Read the model definition and answer for the solid it produces. Units are mm, in the model's axes. A direction names the side the tool comes from. Give positions to 0.01 mm unless a question says otherwise; leave off trailing zeros. Order: outer loops, then holes, each group sorted by start corner. A loop starts at its lowest first (then second) coordinate and runs counter-clockwise, first axis right, second up.
Item 1: Given pin 1 Ø3.5 at (y, z) = (-8, 7) entering from -X (3 decimals); pin 2 Ø8 at (y, z) = (22.5, -2.5) entering from -X; pin 3 Ø6 at (y, z) = (-7, 7) entering from +X; pin 4 Ø10 at (x, z) = (-41.5, -6) entering from +Y, each flat-ended and moving along its own axis, determine where each tip first touches the part or whether it passes through.
Item 2: Find the intervals of material crossed by line 1 along Z through (x, y) = (-64, 7); line 2 along X through (y, z) = (-1.5, 8.25) (3 decimals), in increasing order.
Item 3: The mould has two halves that part along Y. Classify faces 3 (the face through (-49, 0, -12.5)), 4 (the face through (-52.461, -14.202, 0.175)), 5 (the face through (-42.024, 24.806, 5.479)): +Y half, -Y half, draft (parallel to the pull), parting line (faces both ways), or undercut.
Item 4: A cutting plane is placed at C-C (z = 1.75). Write down the section's boundary in (x, y) (3 decimals).
Item 5: Which of the six approach directions +Z, -Z, +X, -X, +Y, -Y give full straight-line access (tool end or side, diameter ignored) to faces 1 (the face through (-63.64, -8.52, 8.66)), 2 (the face through (-29, -37.067, 0))?
Item 6: A cutting plane is placed at A-A (z = -7). State how many separate pieces and enclosed holes the cut face has, plus the area to 3 significant figures.
Item 7: A cutting plane is placed at B-B (y = 6). Write down the section's boundary in (x, z) (3 decimals).
Item 8: A cutting plane is placed at D-D (x = -56). Write down the section's boundary in (y, z), plus the area to 3 significant figures.
from build123d import *

# Parameters (mm, degrees)
BOSS_EXTRUDE1_DEPTH     = 12.5
SKETCH3_R               = 2.25
CUT_EXTRUDE1_DEPTH      = 77.872073504
CUT_EXTRUDE2_DEPTH      = 57.106034184
CUT_EXTRUDE2_DEPTH_BACK = 5
SKETCH5_R               = 2.25
FILLET4_R               = 10


with BuildPart() as part:
    # Sketch1 → Boss-Extrude1 (new, symmetric)
    with BuildSketch(Plane.XY):
        with BuildLine():
            Line((-66.175, -12.5), (-66.175, 12.5))
            Line((-66.175, 12.5), (-50.732755691, 12.5))
            ThreePointArc((-50.732755691, 12.5), (-45.469745991, 25.740332157), (-36.825635638, 37.066630004))
            Line((-36.825635638, 37.066630004), (-25.954333745, 37.066630004))
            ThreePointArc((-25.954333745, 37.066630004), (-45.25, 0), (-25.954333745, -37.066630004))
            Line((-25.954333745, -37.066630004), (-36.825635638, -37.066630004))
            ThreePointArc((-36.825635638, -37.066630004), (-45.469745991, -25.740332157), (-50.732755691, -12.5))
            Line((-50.732755691, -12.5), (-66.175, -12.5))
        make_face()
    extrude(amount=BOSS_EXTRUDE1_DEPTH, both=True)

    # Sketch3 → Cut-Extrude1 (cut, symmetric)
    with BuildSketch(Plane(origin=(0, 0, 0), x_dir=(0, 0, 1), z_dir=(-0.8433914458128852, 0.5372996083468248, 0))):
        with Locations(Location((-7, 0, 0), (0, 0, 90))):
            Circle(SKETCH3_R)
        with Locations(Location((7, 0, 0), (0, 0, 90))):
            Circle(SKETCH3_R)
    cut_extrude1 = extrude(amount=CUT_EXTRUDE1_DEPTH, both=True, mode=Mode.SUBTRACT)

    # Mirror1: Cut-Extrude1 across plane
    add(cut_extrude1.mirror(Plane.ZX), mode=Mode.SUBTRACT)

    # Sketch5 → Cut-Extrude2 (cut, two sides: drawn at the far end of the back side and taken through both)
    with BuildSketch(Plane.ZY.offset(66.175).offset(-CUT_EXTRUDE2_DEPTH_BACK)):
        with Locations(Location((-7, 7, 0), (0, 0, 180))):
            Circle(SKETCH5_R)
        with Locations(Location((7, 7, 0), (0, 0, 180))):
            Circle(SKETCH5_R)
        with Locations(Location((7, -7, 0), (0, 0, 180))):
            Circle(SKETCH5_R)
        with Locations(Location((-7, -7, 0), (0, 0, 180))):
            Circle(SKETCH5_R)
    extrude(amount=CUT_EXTRUDE2_DEPTH + CUT_EXTRUDE2_DEPTH_BACK, mode=Mode.SUBTRACT)

    # Fillet4
    fillet4_edges = [part.edges().sort_by_distance(p)[0] for p in [
        (-36.825635638, -37.066630004, 0),
        (-50.732755691, -12.5, 0),
        (-50.732755691, 12.5, 0),
        (-36.825635638, 37.066630004, 0),
    ]]
    fillet(fillet4_edges, radius=FILLET4_R)


solid = part.part
Response values:
1. pin 1: stops at x = -66.175
1. pin 2: stops at x = -48.88
1. pin 3: stops at x = -44.13
1. pin 4: stops at y = 36.21
2. line 1: z = -12.5 to -9.25, -4.75 to 4.75, 9.25 to 12.5
2. line 2: x = -66.175 to -45.225
3. face 3: draft
3. face 4: -Y half
3. face 5: undercut
4. outline: (-66.175, -12.5) - (-58.041, -12.5) arc R10 cw to (-48.718, -18.886) arc R52.25 ccw to (-40.12, -33.473) arc R10 ccw to (-32.442, -37.067) - (-25.954, -37.067) arc R45.25 cw to (-25.954, 37.067) - (-32.442, 37.067) arc R10 ccw to (-40.12, 33.473) arc R52.25 ccw to (-48.718, 18.886) arc R10 cw to (-58.041, 12.5) - (-66.175, 12.5) - close
5. face 1: -X
5. face 2: +Z, -Z, +X, -X, -Y
6. separate pieces: 3
6. enclosed holes: 0
6. area: 857 mm2
7. outline: (-66.175, -12.5) - (-44.85, -12.5) - (-44.85, 12.5) - (-66.175, 12.5) - (-66.175, 9.016) - (-61.175, 9.016) - (-61.175, 4.984) - (-66.175, 4.984) - (-66.175, -4.984) - (-61.175, -4.984) - (-61.175, -9.016) - (-66.175, -9.016) - close
8. outline: (-12.71, -12.5) - (12.71, -12.5) - (12.71, 12.5) - (-12.71, 12.5) - close
8. area: 636 mm2
